Check sheet for the modelled part. Datum: model origin and axes. Units: mm. A direction names the side the tool comes from. Round coordinates to 2 decimals unless told otherwise and drop trailing zeros. Loops run counter-clockwise (first coordinate to the right, second up) from the corner with the lowest first, then second, coordinate; pieces in that order, holes last. Notation, with made-up numbers: (81.25, 2.5) -> (137.25, 2.5) arc R19 ccw to (137.25, 21.5) -> close; hole circle Ø5 at (27, -30). An arc over 180 degrees is marked (long way). One line per question, with ' | ' between items.
```python
from build123d import *

# Parameters (mm, degrees)
SKETCH1_R           = 23
SKETCH1_R_2         = 3.5
SKETCH1_R_3         = 8
SKETCH1_R_4         = 2.5
BOSS_EXTRUDE1_DEPTH = 5
SKETCH1_3_R         = 8
SKETCH1_3_R_2       = 2.5
BOSS_EXTRUDE2_DEPTH = 32
CHAMFER1_SIZE       = 0.5
CHAMFER2_SIZE       = 0.25
CHAMFER3_SIZE       = 1


with BuildPart() as part:
    # Sketch1 → Boss-Extrude1 (new body)
    # profile 1 of 2: a face of its own
    with BuildSketch(Plane(origin=(0, 0, 0), x_dir=(1, 0, 0), z_dir=(0, 1, 0))):
        with Locations(Location((0, 0, 0), (0, 0, 270))):
            Circle(SKETCH1_R)
        with Locations(Location((0, 15, 0), (0, 0, 270))):
            Circle(SKETCH1_R_2, mode=Mode.SUBTRACT)
        Circle(SKETCH1_R_3, mode=Mode.SUBTRACT)
    # profile 2 of 2: a face of its own
    with BuildSketch(Plane(origin=(0, 0, 0), x_dir=(1, 0, 0), z_dir=(0, 1, 0))):
        Circle(SKETCH1_R_3)
        with Locations(Location((0, 0, 0), (0, 0, 270))):
            Circle(SKETCH1_R_4, mode=Mode.SUBTRACT)
    extrude(amount=BOSS_EXTRUDE1_DEPTH)

    # Sketch1_3 → Boss-Extrude2 (add)
    with BuildSketch(Plane(origin=(0, 0, 0), x_dir=(1, 0, 0), z_dir=(0, 1, 0))):
        with Locations(Location((0, 0, 0), (0, 0, 270))):
            Circle(SKETCH1_3_R)
        with Locations(Location((0, 0, 0), (0, 0, 270))):
            Circle(SKETCH1_3_R_2, mode=Mode.SUBTRACT)
    extrude(amount=BOSS_EXTRUDE2_DEPTH)

    # Chamfer1
    chamfer1_edges = [part.edges().sort_by_distance(p)[0] for p in [
        (0, 32, -8),
    ]]
    chamfer(chamfer1_edges, length=CHAMFER1_SIZE)

    # Chamfer2
    chamfer2_edges = [part.edges().sort_by_distance(p)[0] for p in [
        (0, 5, -23),
        (0, 0, -23),
    ]]
    chamfer(chamfer2_edges, length=CHAMFER2_SIZE)

    # Chamfer3
    chamfer3_edges = [part.edges().sort_by_distance(p)[0] for p in [
        (0, 0, -18.5),
    ]]
    chamfer(chamfer3_edges, length=CHAMFER3_SIZE)


solid = part.part
```
(1) Sectioned sample at A-A, the plane z = 0. Record the cut outline in (x, y), and give its area (3 significant figures).
Answer:
outline: (-23, 0.25) -> (-22.75, 0) -> (-2.5, 0) -> (-2.5, 32) -> (-7.5, 32) -> (-8, 31.5) -> (-8, 5) -> (-22.75, 5) -> (-23, 4.75) -> close; (2.5, 0) -> (22.75, 0) -> (23, 0.25) -> (23, 4.75) -> (22.75, 5) -> (8, 5) -> (8, 31.5) -> (7.5, 32) -> (2.5, 32) -> close | area: 502 mm2
(2) Mould release check, pull along Z, two halves, no side actions. Record for faces 1 (the face through (-2.44, 15.78, -0.54)), 2 (the face through (2, 32, -2)), 3 (the face through (-7.81, 18.06, -1.73)): +Z half, -Z half, draft (parallel to the pull), parting line (faces both ways), or undercut.
Answer:
face 1: undercut | face 2: draft | face 3: parting line
(3) Sectioned sample at C-C, the plane y = 17.5. Record the cut outline in (x, z).
Answer:
outline: circle Ø16 at (0, 0); hole circle Ø5 at (0, 0)
(4) Scan lines: probe 1 along X at (y, z) = (13.5, 0); probe 2 along X at (y, z) = (8, 1); probe 3 along Z at (x, y) = (2, 18). Record each from-to range of solid material in increasing order.
Answer:
probe 1: x = -8 to -2.5, 2.5 to 8 | probe 2: x = -7.94 to -2.29, 2.29 to 7.94 | probe 3: z = -7.75 to -1.5, 1.5 to 7.75
(5) Set-up check for faces 4 (the face through (19.394, 2.468, 12.365)), 5 (the face through (0, 5, 10)): record each of +Z, -Z, +X, -X, +Y, -Y from which the full face is reachable in a straight line by a thin tool's end or side.
Answer:
face 4: +Y, -Y | face 5: +Y
(6) Go/stop test with flat-tipped pins: pin 1 (1 mm diameter, centred on y = 13.5, z = -2.5, fed in from +X); pin 2 (3 mm diameter, centred on x = 7.5, y = 10, fed in from +Z); pin 3 (5.5 mm diameter, centred on x = 0, z = -15, fed in from -Y); pin 4 (12 mm diameter, centred on x = -3, y = 21, fed in from -Z). Record where each tip stops, or that it passes through.
Answer:
pin 1: stops at x = 7.75 | pin 2: stops at z = 5.29 | pin 3: passes through | pin 4: stops at z = -8
(7) Sectioned sample at B-B, the plane x = 0. Record the cut outline in (y, z), and give its area (3 significant figures).
Answer:
outline: (0, -22.75) -> (0.25, -23) -> (4.75, -23) -> (5, -22.75) -> (5, -18.5) -> (1, -18.5) -> (0, -19.5) -> close; (0, -10.5) -> (1, -11.5) -> (5, -11.5) -> (5, -8) -> (31.5, -8) -> (32, -7.5) -> (32, -2.5) -> (0, -2.5) -> close; (0, 2.5) -> (32, 2.5) -> (32, 7.5) -> (31.5, 8) -> (5, 8) -> (5, 22.75) -> (4.75, 23) -> (0.25, 23) -> (0, 22.75) -> close | area: 466 mm2
